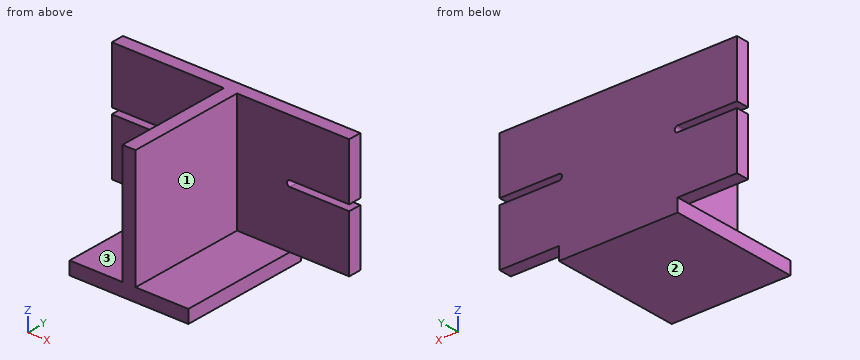
```python
from build123d import *

# Parameters (mm, degrees)
BOSS_EXTRU_1_DEPTH = 22
ESQUISSE2_W        = 22
ESQUISSE2_H        = 200
BOSS_EXTRU_2_DEPTH = 200
ESQUISSE3_W        = 200
ESQUISSE3_H        = 22
BOSS_EXTRU_3_DEPTH = 222


with BuildPart() as part:
    # Esquisse1 → Boss.-Extru.1 (new body)
    with BuildSketch(Plane(origin=(0, 0, 0), x_dir=(1, 0, 0), z_dir=(0, 1, 0))):
        with BuildLine():
            Line((0, 0), (0, -200))
            Line((0, -200), (-200, -200))
            Line((-200, -200), (-200, -105))
            Line((-200, -105), (-100, -105))
            ThreePointArc((-100, -105), (-95, -100), (-100, -95))
            Line((-100, -95), (-200, -95))
            Line((-200, -95), (-200, 0))
            Line((-200, 0), (0, 0))
        make_face()
    boss_extru_1 = extrude(amount=BOSS_EXTRU_1_DEPTH)

    # Symétrie1: Boss.-Extru.1 across plane
    add(boss_extru_1.mirror(Plane(origin=(0, 22, 0), x_dir=(0, 0, 1), z_dir=(-1, 0, 0))))

    # Esquisse2 → Boss.-Extru.2 (add)
    with BuildSketch(Plane.XZ):
        with Locations((0, 100)):
            Rectangle(ESQUISSE2_W, ESQUISSE2_H)
    extrude(amount=BOSS_EXTRU_2_DEPTH)

    # Esquisse3 → Boss.-Extru.3 (add)
    with BuildSketch(Plane(origin=(0, 22, 0), x_dir=(1, 0, 0), z_dir=(0, 1, 0))):
        with Locations((0, 11)):
            Rectangle(ESQUISSE3_W, ESQUISSE3_H)
    extrude(amount=-BOSS_EXTRU_3_DEPTH)


solid = part.part
```
Build history of the part. All positions in model axes, mm. Face numbers are marked on the shaded views. A direction names the side the tool comes from. Round coordinates to 2 decimals unless told otherwise and drop trailing zeros. Write each loop counter-clockwise with the first axis right and the second up, starting at its lowest first coordinate (ties: lowest second). Pieces come first, ordered by that corner, then holes.
1) 3-axis set-ups, long thin cutter, end or side, ignore diameter. For the marked faces 1, 2 and 3: which of +Z, -Z, +X, -X, +Y, -Y reach the whole face in a straight line?
2) Band-saw the part on D-D, the plane x = -21.5. List the corners of the cut face in (y, z).
3) Pin check, flat tips, straight feed: pin 1 (5 mm diameter, centred on y = -161, z = 96, fed in from +X); pin 2 (11 mm diameter, centred on x = 130, y = 6.5, fed in from -Z); pin 3 (6 mm diameter, centred on x = -78, y = -91, fed in from +Z). Stop position of each tip, or through.
4) Band-saw the part on B-B, the plane z = 100. List the corners of the cut face in (x, y).
5) Drill centre lines: probe 1 along Y at (x, z) = (35, 65.5); probe 2 along Z at (x, y) = (74.5, -26.5); probe 3 along X at (y, z) = (-59, -10.5). Where is each one in solid material? Low to high.
6) Band-saw the part on A-A, the plane x = 133.5. List the corners of the cut face in (y, z).
7) Band-saw the part on C-C, the plane y = -87. List the corners of the cut face in (x, z), and give its area (3 significant figures).
Ans:
1. face 1: +Z, +X, -Y
1. face 2: -Z, +X, -X, +Y, -Y
1. face 3: +Z, -X, -Y
2. outline: (-200, -22) - (22, -22) - (22, 200) - (0, 200) - (0, 0) - (-200, 0) - close
3. pin 1: stops at x = 11
3. pin 2: stops at z = 0
3. pin 3: stops at z = 0
4. outline: (-95, 0) - (-11, 0) - (-11, -200) - (11, -200) - (11, 0) - (95, 0) - (95, 22) - (-95, 22) - close
5. probe 1: y = 0 to 22
5. probe 2: z = -22 to 0
5. probe 3: x = -100 to 100
6. outline: (0, 0) - (22, 0) - (22, 95) - (0, 95) - close; (0, 105) - (22, 105) - (22, 200) - (0, 200) - close
7. outline: (-100, -22) - (100, -22) - (100, 0) - (11, 0) - (11, 200) - (-11, 200) - (-11, 0) - (-100, 0) - close
7. area: 8,800 mm2
